For this review, use the dimensioned drawing (mm, ordinates from the lowest corner) and the shaded views. Give positions to 0.01 mm unless a question says otherwise; leave off trailing zeros. Order: outer loops, then holes, each group sorted by start corner. A loop starts at its lowest first (then second) coordinate and runs counter-clockwise, first axis right, second up.
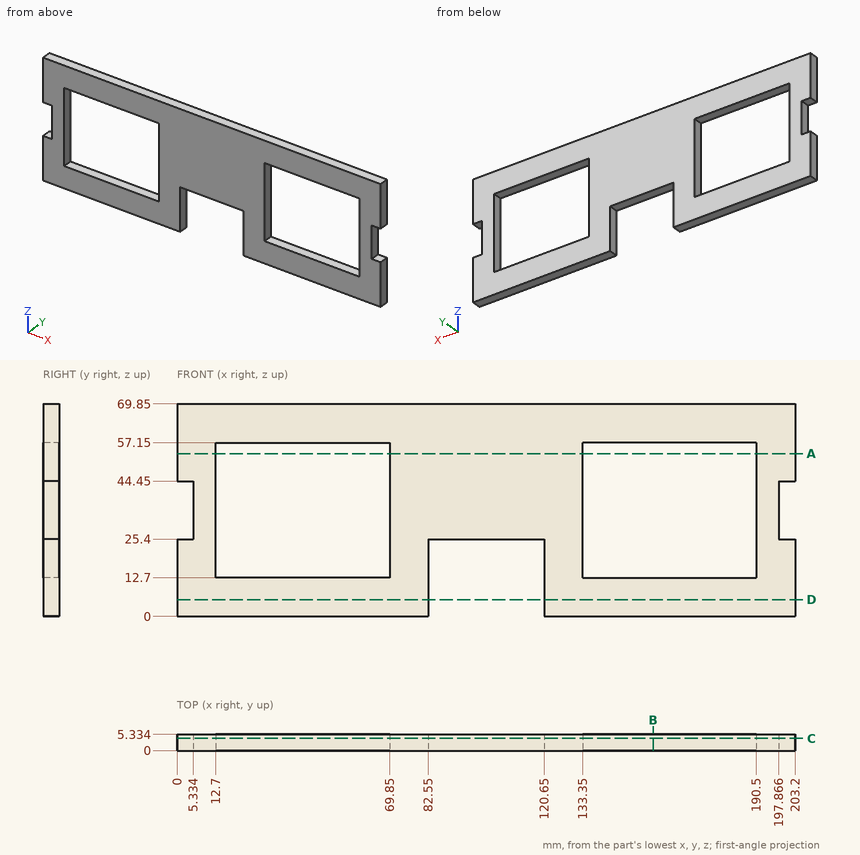
1. Take a section at B-B (x = 156.5). State the section outline as (y, z) points, then the cut area to 3 significant figures.
Recorded:
outline: (0, 0) - (5.33, 0) - (5.33, 12.7) - (0, 12.7) - close; (0, 57.15) - (5.33, 57.15) - (5.33, 69.85) - (0, 69.85) - close
area: 135 mm2
2. Take a section at D-D (z = 5.5). State the section outline as (x, y) points.
Recorded:
outline: (0, 0) - (82.55, 0) - (82.55, 5.33) - (0, 5.33) - close; (120.65, 0) - (203.2, 0) - (203.2, 5.33) - (120.65, 5.33) - close
3. For line 1 along X through (y, z) = (3.75, 49.5); line 2 along X through (y, z) = (3.05, 21); line 3 along X through (y, z) = (0.4, 40), list the stretches that pass through material, from the lowest coordinate up.
Recorded:
line 1: x = 0 to 12.7, 69.85 to 133.35, 190.5 to 203.2
line 2: x = 0 to 12.7, 69.85 to 82.55, 120.65 to 133.35, 190.5 to 203.2
line 3: x = 5.33 to 12.7, 69.85 to 133.35, 190.5 to 197.87
4. For pin 1 (1 mm diameter, centred on y = 1.5, z = 31.5, fed in from -X); pin 2 (2 mm diameter, centred on x = 108.5, y = 0.5, fed in from -Z), all flat-tipped, find the tip position at first contact; note any pin that passes through.
Recorded:
pin 1: stops at x = 5.33
pin 2: stops at z = 25.4
5. Take a section at C-C (y = 4). State the section outline as (x, z) points, then the cut area to 3 significant figures.
Recorded:
outline: (0, 0) - (82.55, 0) - (82.55, 25.4) - (120.65, 25.4) - (120.65, 0) - (203.2, 0) - (203.2, 25.4) - (197.87, 25.4) - (197.87, 44.45) - (203.2, 44.45) - (203.2, 69.85) - (0, 69.85) - (0, 44.45) - (5.33, 44.45) - (5.33, 25.4) - (0, 25.4) - close; hole (12.7, 12.7) - (69.85, 12.7) - (69.85, 57.15) - (12.7, 57.15) - close; hole (133.35, 12.7) - (190.5, 12.7) - (190.5, 57.15) - (133.35, 57.15) - close
area: 7,940 mm2
6. Take a section at A-A (z = 53.5). State the section outline as (x, y) points.
Recorded:
outline: (0, 0) - (12.7, 0) - (12.7, 5.33) - (0, 5.33) - close; (69.85, 0) - (133.35, 0) - (133.35, 5.33) - (69.85, 5.33) - close; (190.5, 0) - (203.2, 0) - (203.2, 5.33) - (190.5, 5.33) - close
